```python
from build123d import *

# Parameters (mm, degrees)
EXTRUDE_1_DEPTH     = 3
SKETCH_2_W          = 10
SKETCH_2_H          = 3
CUT_EXTRUDE_1_DEPTH = 3


with BuildPart() as part:
    # 草圖1 → 填料-伸長1 (new body)
    with BuildSketch(Plane.XY):
        Polygon((49.262888429, -24.540240663), (49.262888429, -21.540240663), (39.262888429, -21.540240663), (39.262888429, -24.540240663), (25.262888429, -24.540240663), (25.262888429, -21.540240663), (15.262888429, -21.540240663), (15.262888429, -24.540240663), (1.262888429, -24.540240663), (1.262888429, -21.540240663), (-8.737111571, -21.540240663), (-8.737111571, -24.540240663), (-22.737111571, -24.540240663), (-22.737111571, -21.540240663), (-32.737111571, -21.540240663), (-32.737111571, -24.540240663), (-41.737111571, -24.540240663), (-41.737111571, -9.540240663), (-38.737111571, -9.540240663), (-38.737111571, 0.459759337), (-41.737111571, 0.459759337), (-41.737111571, 15.459759337), (-32.737111571, 15.459759337), (-32.737111571, 12.459759337), (-22.737111571, 12.459759337), (-22.737111571, 15.459759337), (-8.737111571, 15.459759337), (-8.737111571, 12.459759337), (1.262888429, 12.459759337), (1.262888429, 15.459759337), (15.262888429, 15.459759337), (15.262888429, 12.459759337), (25.262888429, 12.459759337), (25.262888429, 15.459759337), (39.262888429, 15.459759337), (39.262888429, 12.459759337), (49.262888429, 12.459759337), (49.262888429, 15.459759337), (58.262888429, 15.459759337), (58.262888429, 0.459759337), (55.262888429, 0.459759337), (55.262888429, -9.540240663), (58.262888429, -9.540240663), (58.262888429, -24.540240663), align=None)
    extrude(amount=EXTRUDE_1_DEPTH)

    # 草圖2 → 除料-伸長1 (cut)
    with BuildSketch(Plane.XY.offset(3)):
        with Locations((8.262888429, 3.959759337)):
            Rectangle(SKETCH_2_W, SKETCH_2_H)
    extrude(amount=-CUT_EXTRUDE_1_DEPTH, mode=Mode.SUBTRACT)


solid = part.part
```
Here's how the part is built. I have some questions about the finished solid (model axes, mm). A direction names the side the tool comes from. Coordinates: 2 decimals unless noted, no trailing zeros. Write each loop counter-clockwise with the first axis right and the second up, starting at its lowest first coordinate (ties: lowest second). Pieces come first, ordered by that corner, then holes. Notation, with made-up numbers: (44, 24) -> (54, 24) arc R17 cw to (54, 42) -> close; hole circle Ø6 at (56.5, -1). An arc over 180 degrees is marked (long way). Use a Markdown table: item, result. Add a question column.
(1) For faces 1 (the flat face through (8, 2.46, 2)), 2 (the flat face through (25.263, 14, 1)), 3 (the flat face through (-37, -24.54, 1)), 4 (the flat face through (44, -21.54, 1)), which set-ups out of +Z, -Z, +X, -X, +Y, -Y let a thin tool reach every point of the face, with its end or its side?
(2) If we section it at B-B, the plane y = -2: Write out the boundary of the cut face in (x, z).
(3) I'm going to push flat-ended pins straight in: P1, Ø0.9, axis at y = -3, z = 2, coming from the +X side; P2, Ø0.9, axis at x = 42.5, z = 2, coming from the -Y side; P3, Ø1.5, axis at x = 44, z = 1, coming from the +Y side. Where does each tip first touch, or does it pass through?
(4) Please list where these lines run through material, in increasing order: line 1 (X direction, y = 3.5, z = 0.35); line 2 (Y direction, x = 9.5, z = 0.95); line 3 (X direction, y = -8, z = 1.65).
(5) If we section it at C-C, the plane x = 18.5: Write out the boundary of the cut face in (y, z).
(6) We'd pull the mould along X, two halves only. Please class faces 5 (the flat face through (49.263, 14, 1)), 6 (the flat face through (-41.737, -17, 1)), 7 (the flat face through (58.263, -17, 1)), 8 (the flat face through (8, -24.54, 1)): +X half, -X half, draft (parallel to the pull), parting line (faces both ways), or undercut.
(7) If we section it at A-A, the plane x = 8: Write out the boundary of the cut face in (y, z), and give its area (3 significant figures).
Outcome:
| question | item | result |
|---|---|---|
| 1 | face 1 | +Z, -Z |
| 1 | face 2 | +Z, -Z, +Y |
| 1 | face 3 | +Z, -Z, +X, -X, -Y |
| 1 | face 4 | +Z, -Z, -Y |
| 2 | outline | (-38.74, 0) -> (55.26, 0) -> (55.26, 3) -> (-38.74, 3) -> close |
| 3 | P1 | stops at x = 55.26 |
| 3 | P2 | stops at y = -21.54 |
| 3 | P3 | stops at y = 12.46 |
| 4 | line 1 | x = -41.74 to 3.26, 13.26 to 58.26 |
| 4 | line 2 | y = -24.54 to 2.46, 5.46 to 15.46 |
| 4 | line 3 | x = -38.74 to 55.26 |
| 5 | outline | (-21.54, 0) -> (12.46, 0) -> (12.46, 3) -> (-21.54, 3) -> close |
| 6 | face 5 | undercut |
| 6 | face 6 | -X half |
| 6 | face 7 | +X half |
| 6 | face 8 | draft |
| 7 | outline | (-24.54, 0) -> (2.46, 0) -> (2.46, 3) -> (-24.54, 3) -> close; (5.46, 0) -> (15.46, 0) -> (15.46, 3) -> (5.46, 3) -> close |
| 7 | area | 111 mm^2 |
